The model under review builds one solid part; all positions refer to its coordinate system, in mm. A direction names the side the tool comes from. Coordinates: 2 decimals unless noted, no trailing zeros. Write each loop counter-clockwise with the first axis right and the second up, starting at its lowest first coordinate (ties: lowest second). Pieces come first, ordered by that corner, then holes.
```python
from build123d import *

# Parameters (mm, degrees)
SKETCH1_R           = 10
BOSS_EXTRUDE1_DEPTH = 70
SKETCH2_R           = 2
CUT_EXTRUDE1_DEPTH  = 60
FILLET1_R           = 2
CUT_EXTRUDE2_START  = -5
SKETCH4_R           = 2
CUT_EXTRUDE2_DEPTH  = 5


with BuildPart() as part:
    # Sketch1 → Boss-Extrude1 (new body)
    with BuildSketch(Plane(origin=(0, 0, 0), x_dir=(1, 0, 0), z_dir=(0, 1, 0))):
        with Locations(Location((0, 0, 0), (0, 0, 270))):
            Circle(SKETCH1_R)
    extrude(amount=BOSS_EXTRUDE1_DEPTH)

    # Sketch2 → Cut-Extrude1 (cut)
    with BuildSketch(Plane(origin=(0, 70, 0), x_dir=(1, 0, 0), z_dir=(0, 1, 0))):
        with Locations(Location((0, 0, 0), (0, 0, 270))):
            Circle(SKETCH2_R)
    extrude(amount=-CUT_EXTRUDE1_DEPTH, mode=Mode.SUBTRACT)

    # Fillet1
    fillet1_edges = [part.edges().sort_by_distance(p)[0] for p in [
        (0, 0, -10),
        (0, 70, -10),
    ]]
    fillet(fillet1_edges, radius=FILLET1_R)

    # Sketch4 → Cut-Extrude2 (cut)
    with BuildSketch(Plane.XZ.offset(CUT_EXTRUDE2_START)):
        with Locations(Location((0, 0, 0), (0, 0, 90))):
            Circle(SKETCH4_R)
    extrude(amount=CUT_EXTRUDE2_DEPTH, mode=Mode.SUBTRACT)


solid = part.part
```
Item 1: Take a section at A-A, the plane z = 0. Write out the cut boundary in (x, y), plus the area to 3 significant figures.
Solved:
outline: (-10, 2) arc R2 ccw to (-8, 0) - (-2, 0) - (-2, 5) - (2, 5) - (2, 0) - (8, 0) arc R2 ccw to (10, 2) - (10, 68) arc R2 ccw to (8, 70) - (2, 70) - (2, 10) - (-2, 10) - (-2, 70) - (-8, 70) arc R2 ccw to (-10, 68) - close
area: 1,140 mm2
Item 2: Mouldability with a two-part tool opening along X and no side actions: class faces 4 (the face through (-9.76, 34.54, -2.17)), 5 (the face through (0, 10, 0)), 6 (the face through (-2, 0, 2)) as pulls with the +X half, pulls with the -X half, needs draft (parallel to the pull), parting line crosses it, or undercut.
Solved:
face 4: parting line crosses it
face 5: undercut
face 6: needs draft
Item 3: Machinability: for faces 1 (the face through (0, 5, 0)), 2 (the face through (-2, 70, 2)), 3 (the face through (-2, 40, 0)), which of the approach directions +Z, -Z, +X, -X, +Y, -Y give a long, thin tool a straight path to every point of the face, cutting with its end or side? Answer none if there is none.
Solved:
face 1: -Y
face 2: +Z, -Z, +X, -X, +Y
face 3: +Y
Item 4: To check wall thickness, follow line 1 along X through (y, z) = (53.5, 0); line 2 along X through (y, z) = (58.5, -1.75); line 3 along Z through (x, y) = (-0.75, 39). State the ranges of each line that lie inside material, in increasing order.
Solved:
line 1: x = -10 to -2, 2 to 10
line 2: x = -9.85 to -0.97, 0.97 to 9.85
line 3: z = -9.97 to -1.85, 1.85 to 9.97
Item 5: Take a section at B-B, the plane x = 0. Write out the cut boundary in (y, z).
Solved:
outline: (0, -8) arc R2 ccw to (2, -10) - (68, -10) arc R2 ccw to (70, -8) - (70, -2) - (10, -2) - (10, 2) - (70, 2) - (70, 8) arc R2 ccw to (68, 10) - (2, 10) arc R2 ccw to (0, 8) - (0, 2) - (5, 2) - (5, -2) - (0, -2) - close
Item 6: For pin 1 (3 mm diameter, centred on x = 6.5, z = -2.5, fed in from -Y); pin 2 (6 mm diameter, centred on x = 4, y = 63, fed in from -Z); pin 3 (3 mm diameter, centred on y = 13.5, z = 2.5, fed in from -X); pin 4 (3 mm diameter, centred on x = -2, y = 54, fed in from -Z), all flat-tipped, find the tip position at first contact; note any pin that passes through.
Solved:
pin 1: stops at y = 0
pin 2: stops at z = -9.95
pin 3: stops at x = -9.95
pin 4: stops at z = -9.99
Item 7: Take a section at C-C, the plane y = 61.5. Write out the cut boundary in (x, z).
Solved:
outline: circle Ø20 at (0, 0); hole circle Ø4 at (0, 0)
